```python
from build123d import *

# Parameters (mm, degrees)
SKETCH_1_R               = 80
EXTRUDE_1_DEPTH          = 12
SKETCH_1_3_R             = 45
SKETCH_1_3_R_2           = 25
EXTRUDE_2_DEPTH          = 33
CUT_EXTRUDE_2_DEPTH      = 118.851601601
CUT_EXTRUDE_2_DEPTH_BACK = 118.851601601
SKETCH_1_4_R             = 25
SKETCH_3_R               = 7.5
CUT_EXTRUDE_3_DEPTH      = 116.06954419
CUT_EXTRUDE_4_DEPTH      = 118.851601601
CUT_EXTRUDE_4_DEPTH_BACK = 118.851601601
SKETCH_4_R               = 3.25
EXTRUDE_3_DEPTH          = 21
FILLET_1_R               = 10
CUT_EXTRUDE_START        = 73.821646461
CUT_EXTRUDE_5_DEPTH      = 7.178353539
CUT_EXTRUDE_START_2      = 16
CUT_EXTRUDE_5_2_DEPTH    = 13
CUT_EXTRUDE_9_REACH      = 119.852
CUT_EXTRUDE_9_END_RADIUS = 80


with BuildPart() as part:
    # 草图1 → 凸台-拉伸1 (new body)
    with BuildSketch(Plane(origin=(0, 0, 0), x_dir=(1, 0, 0), z_dir=(0, 1, 0))):
        with Locations(Location((0, 0, 0), (0, 0, 270))):
            Circle(SKETCH_1_R)
    extrude(amount=EXTRUDE_1_DEPTH)

    # 草图1<3> → 凸台-拉伸2 (add)
    with BuildSketch(Plane(origin=(0, 0, 0), x_dir=(1, 0, 0), z_dir=(0, 1, 0))):
        with Locations(Location((0, 0, 0), (0, 0, 270))):
            Circle(SKETCH_1_3_R)
        with Locations(Location((0, 0, 0), (0, 0, 270))):
            Circle(SKETCH_1_3_R_2, mode=Mode.SUBTRACT)
    extrude(amount=EXTRUDE_2_DEPTH)

    # 草图1<4> → 切除-拉伸2 (cut, two sides: drawn at the far end of the back side and taken through both)
    with BuildSketch(Plane(origin=(0, 0, 0), x_dir=(1, 0, 0), z_dir=(0, 1, 0)).offset(-CUT_EXTRUDE_2_DEPTH_BACK)):
        with Locations(Location((0, 0, 0), (0, 0, 270))):
            Circle(SKETCH_1_4_R)
    extrude(amount=CUT_EXTRUDE_2_DEPTH + CUT_EXTRUDE_2_DEPTH_BACK, mode=Mode.SUBTRACT)

    # 草图3 → 切除-拉伸3 (cut, through all)
    with BuildSketch(Plane(origin=(0, 12, 0), x_dir=(1, 0, 0), z_dir=(0, 1, 0))):
        with Locations(Location((0, 60, 0), (0, 0, 270))):
            Circle(SKETCH_3_R)
        with Locations(Location((0, -60, 0), (0, 0, 270))):
            Circle(SKETCH_3_R)
    extrude(amount=-CUT_EXTRUDE_3_DEPTH, mode=Mode.SUBTRACT)

    # 草图4 → 切除-拉伸4 (cut, two sides: drawn at the far end of the back side and taken through both)
    with BuildSketch(Plane.XY.offset(-CUT_EXTRUDE_4_DEPTH_BACK)):
        with Locations((0, 23)):
            Circle(SKETCH_4_R)
    extrude(amount=CUT_EXTRUDE_4_DEPTH + CUT_EXTRUDE_4_DEPTH_BACK, mode=Mode.SUBTRACT)

    # 草图6 → 凸台-拉伸3 (add)
    with BuildSketch(Plane(origin=(0, 12, 0), x_dir=(1, 0, 0), z_dir=(0, 1, 0))):
        with BuildLine():
            ThreePointArc((42.426406871, 15), (44.351935184, 7.609589043), (45, 0))
            Line((45, 0), (80, 0))
            ThreePointArc((80, 0), (79.64450219, 7.533476681), (78.581168228, 15))
            Line((78.581168228, 15), (42.426406871, 15))
        make_face()
        with BuildLine():
            Line((80, 0), (45, 0))
            ThreePointArc((45, 0), (44.351935184, -7.609589043), (42.426406871, -15))
            Line((42.426406871, -15), (78.581168228, -15))
            ThreePointArc((78.581168228, -15), (79.64450219, -7.533476681), (80, 0))
        make_face()
    extrude(amount=EXTRUDE_3_DEPTH)

    # 圆角1
    fillet_1_edges = [part.edges().sort_by_distance(p)[0] for p in [
        (42.426406871, 22.5, 15),
        (42.426406871, 22.5, -15),
    ]]
    fillet(fillet_1_edges, radius=FILLET_1_R)

    # 切除-拉伸5: read off the stored shape, not the designer's step
    # 切除-拉伸5 outline → 切除-拉伸5 (cut)
    with BuildSketch(Plane(origin=(0, 0, 0), x_dir=(0, 0, -1), z_dir=(1, 0, 0)).offset(CUT_EXTRUDE_START)):
        with BuildLine():
            add(Edge.make_bspline(
                [(-5.338983078, 22.5), (-5.338983078, 21.088703826), (-4.759775949, 19.709126885), (-2.789970131, 17.739694705), (-1.396039111, 17.161767053), (1.390295629, 17.160268335), (2.776177958, 17.726669289), (4.77067497, 19.719260807), (5.338481287, 21.104216537), (5.339484178, 23.891942041), (4.762391942, 25.286161316), (2.795373983, 27.256990244), (1.41465075, 27.837582336), (-1.404057944, 27.840378566), (-2.786176586, 27.262719547), (-4.758291506, 25.293732162), (-5.338983078, 23.911296174), (-5.338983078, 22.5)],
                knots=[0, 0, 0, 0, 0.125, 0.125, 0.25, 0.25, 0.375, 0.375, 0.5, 0.5, 0.625, 0.625, 0.75, 0.75, 0.875, 0.875, 1, 1, 1, 1], degree=3))
        make_face()
    extrude(amount=CUT_EXTRUDE_5_DEPTH, mode=Mode.SUBTRACT)

    # Cut-Extrude 5 2 outline → Cut-Extrude 5 2 (add)
    with BuildSketch(Plane(origin=(0, 0, 0), x_dir=(1, 0, 0), z_dir=(0, 1, 0)).offset(CUT_EXTRUDE_START_2)):
        with BuildLine():
            ThreePointArc((73.821646533, -5.338983493), (74, -1.64e-07), (73.821646555, 5.338983165))
            Line((73.821646555, 5.338983165), (73.821646533, -5.338983493))
        make_face()
    extrude(amount=CUT_EXTRUDE_5_2_DEPTH)

    # 切除-拉伸9: up to this cylinder (the profile starts inside it)
    cut_extrude_9_end = Plane(origin=(-6, 22.5, 0), z_dir=(0, -1, 0)) * Cylinder(CUT_EXTRUDE_9_END_RADIUS, 400.704, mode=Mode.PRIVATE)
    # 草图8<6> → 切除-拉伸9 (cut, up to the surface)
    with BuildSketch(Plane(origin=(0, 0, 0), x_dir=(0, 0, -1), z_dir=(1, 0, 0)), mode=Mode.PRIVATE) as cut_extrude_9_sk1:
        with BuildLine():
            Line((0, 20.21230794), (0, 22.5))
            Line((0, 22.5), (0, 24.78769206))
            ThreePointArc((0, 24.78769206), (-2.28769206, 22.5), (0, 20.21230794))
        make_face()
    cut_extrude_9_tool1 = extrude(cut_extrude_9_sk1.sketch, amount=CUT_EXTRUDE_9_REACH, mode=Mode.PRIVATE) & cut_extrude_9_end
    add(cut_extrude_9_tool1.solids().sort_by_distance((0, 22.5, 0.970927))[0], mode=Mode.SUBTRACT)
    # 草图8<6> → 切除-拉伸9 (cut, up to the surface)
    with BuildSketch(Plane(origin=(0, 0, 0), x_dir=(0, 0, -1), z_dir=(1, 0, 0)), mode=Mode.PRIVATE) as cut_extrude_9_sk2:
        with BuildLine():
            Line((0, 24.78769206), (0, 22.5))
            Line((0, 22.5), (0, 20.21230794))
            ThreePointArc((0, 20.21230794), (1.617642569, 20.882357431), (2.28769206, 22.5))
            ThreePointArc((2.28769206, 22.5), (1.617642569, 24.117642569), (0, 24.78769206))
        make_face()
    cut_extrude_9_tool2 = extrude(cut_extrude_9_sk2.sketch, amount=CUT_EXTRUDE_9_REACH, mode=Mode.PRIVATE) & cut_extrude_9_end
    add(cut_extrude_9_tool2.solids().sort_by_distance((0, 22.5, -0.970927))[0], mode=Mode.SUBTRACT)
    # 草图8<6> → 切除-拉伸9 (cut, up to the surface)
    with BuildSketch(Plane(origin=(0, 0, 0), x_dir=(0, 0, -1), z_dir=(1, 0, 0)), mode=Mode.PRIVATE) as cut_extrude_9_sk3:
        with BuildLine():
            Line((0, 20.21230794), (0, 22.5))
            Line((0, 22.5), (0, 24.78769206))
            ThreePointArc((0, 24.78769206), (-2.28769206, 22.5), (0, 20.21230794))
        make_face()
    cut_extrude_9_tool3 = extrude(cut_extrude_9_sk3.sketch, amount=CUT_EXTRUDE_9_REACH, mode=Mode.PRIVATE) & cut_extrude_9_end
    add(cut_extrude_9_tool3.solids().sort_by_distance((0, 22.5, 0.970927))[0], mode=Mode.SUBTRACT)
    # 草图8<6> → 切除-拉伸9 (cut, up to the surface)
    with BuildSketch(Plane(origin=(0, 0, 0), x_dir=(0, 0, -1), z_dir=(1, 0, 0)), mode=Mode.PRIVATE) as cut_extrude_9_sk4:
        with BuildLine():
            Line((0, 24.78769206), (0, 22.5))
            Line((0, 22.5), (0, 20.21230794))
            ThreePointArc((0, 20.21230794), (1.617642569, 20.882357431), (2.28769206, 22.5))
            ThreePointArc((2.28769206, 22.5), (1.617642569, 24.117642569), (0, 24.78769206))
        make_face()
    cut_extrude_9_tool4 = extrude(cut_extrude_9_sk4.sketch, amount=CUT_EXTRUDE_9_REACH, mode=Mode.PRIVATE) & cut_extrude_9_end
    add(cut_extrude_9_tool4.solids().sort_by_distance((0, 22.5, -0.970927))[0], mode=Mode.SUBTRACT)


solid = part.part
```
CAD build for the part. Positions are in the model's coordinates, mm. A direction names the side the tool comes from. Coordinates: 2 decimals unless noted, no trailing zeros. Order: outer loops, then holes, each group sorted by start corner. A loop starts at its lowest first (then second) coordinate and runs counter-clockwise, first axis right, second up. Notation, with made-up numbers: (63, 27.5) -> (88, 27.5) arc R20 cw to (88, 50.5) -> close; hole circle Ø7 at (52.25, 46.25). An arc over 180 degrees is marked (long way). Use one line per item in the form item = value. Start each with the question number.
1) Drill centre lines: L1, parallel to Z at x = 0, y = 19; L2, parallel to X at y = 15, z = 0.5 (3 decimals); L3, parallel to Y at x = 0, z = 36. Where is each one in solid material? Low to high. Write a range as [from, to].
2) Band-saw the part on A-A on x = 0. Give the cut face in (y, z), then the cut area to 3 significant figures.
3) Tool access for faces 1 (the cylindrical face through (-44.97, 22.35, -1.68)), 2 (the flat face through (64, 22, -15)), 3 (the cylindrical face through (-0.705, 19.827, 34.752)), 4 (the cylindrical face through (43.702, 22.647, 16.512)): list every direction of +Z, -Z, +X, -X, +Y, -Y with a clear straight run to the whole face (end or side of a thin tool).
4) Drop flat-ended pins along their axis: pin 1 (10.5 mm diameter, centred on x = 0, y = 23, fed in from +Z); pin 2 (3 mm diameter, centred on x = 30.5, y = 21.5, fed in from +Z); pin 3 (10 mm diameter, centred on x = 21.5, y = 27.5, fed in from +Z). Give the stop position or say it passes through.
5) Band-saw the part on C-C on z = 60. Give the cut face in (x, y).
6) Band-saw the part on B-B on y = 14. Give the cut face in (x, z), then the cut area to 3 significant figures.
7) Band-saw the part on D-D on x = 65.5. Give the cut face in (y, z).
8) Pull direction Z, two halves, no side cores. Call faces 5 (the flat face through (64, 22, 15)), 6 (the cylindrical face through (5.1, 6.1, -65.5)), 7 (the cylindrical face through (-0.705, 19.827, -35.036)): +Z half, -Z half, draft (parallel to the pull), parting line (faces both ways), or undercut.
Entries:
q1.L1 = [-45, -25], [25, 45]
q1.L2 = [-44.997, -24.995], [24.995, 79.998]
q1.L3 = [0, 19.75], [26.25, 33]
q2.outline = (0, -80) -> (12, -80) -> (12, -67.5) -> (0, -67.5) -> close; (0, -52.5) -> (12, -52.5) -> (12, -45) -> (19.75, -45) -> (19.75, -25) -> (0, -25) -> close; (0, 25) -> (19.75, 25) -> (19.75, 45) -> (12, 45) -> (12, 52.5) -> (0, 52.5) -> close; (0, 67.5) -> (12, 67.5) -> (12, 80) -> (0, 80) -> close; (26.25, -45) -> (33, -45) -> (33, -25) -> (26.25, -25) -> close; (26.25, 25) -> (33, 25) -> (33, 45) -> (26.25, 45) -> close
q2.area = 1,540 mm2
q3.face_1 = +Y
q3.face_2 = -Z, +X, +Y
q3.face_3 = +Z, -Z
q3.face_4 = +Z, +X, +Y
q4.pin_1 = 45
q4.pin_2 = 34.41
q4.pin_3 = 41.87
q5.outline = (-52.92, 0) -> (-7.5, 0) -> (-7.5, 12) -> (-52.92, 12) -> close; (7.5, 0) -> (52.92, 0) -> (52.92, 12) -> (7.5, 12) -> close
q6.outline = (40.08, -20.45) arc R10 cw to (48.99, -15) -> (78.58, -15) arc R80 ccw to (78.58, 15) -> (48.99, 15) arc R10 cw to (40.08, 20.45) arc R45 ccw (long way) to start; hole circle Ø50 at (0, 0)
q6.area = 5,470 mm2
q7.outline = (0, -45.93) -> (12, -45.93) -> (12, -15) -> (33, -15) -> (33, 15) -> (12, 15) -> (12, 45.93) -> (0, 45.93) -> close; hole circle Ø4.58 at (22.5, 0)
q8.face_5 = +Z half
q8.face_6 = undercut
q8.face_7 = draft
